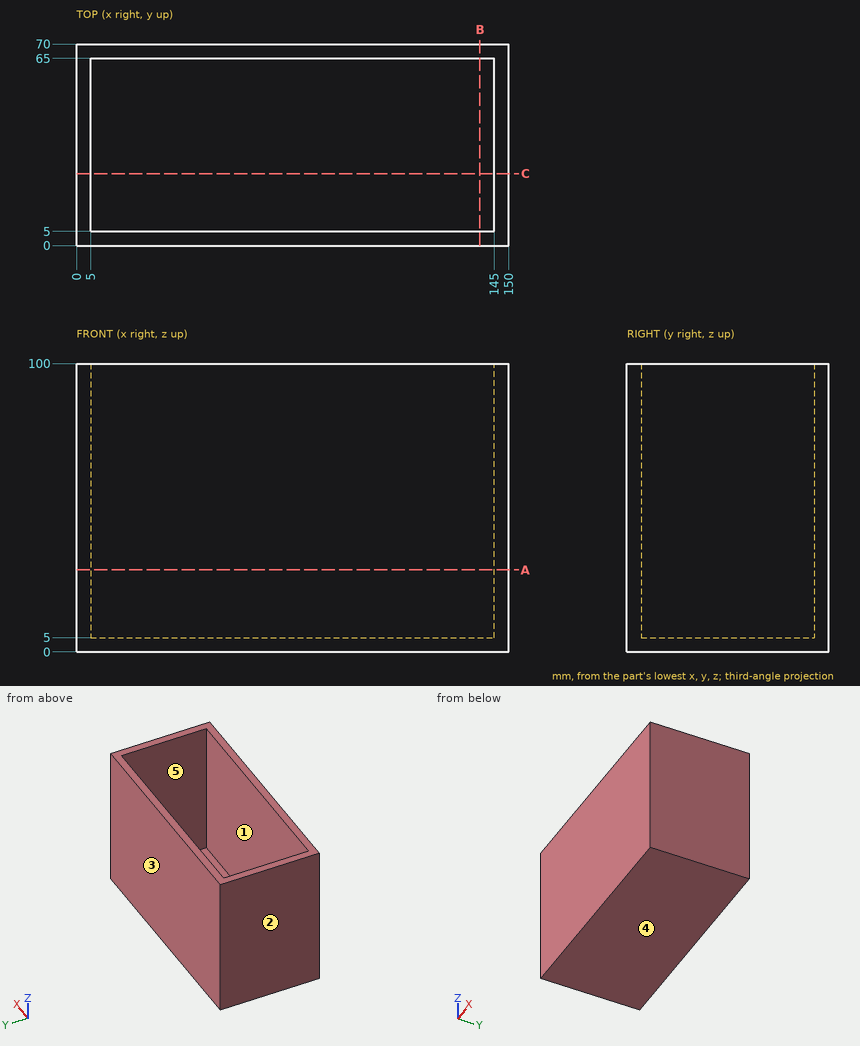
Geometry check sheet. Reference: drawing and pictorial views, mm from the part's lowest x, y, z. A direction names the side the tool comes from. Round coordinates to 2 decimals unless told otherwise and drop trailing zeros. Loops run counter-clockwise (first coordinate to the right, second up) from the corner with the lowest first, then second, coordinate; pieces in that order, holes last.
1. Gauge pin test, flat ends, axial feed: pin 1 Ø10 at (x, y) = (24.5, 17.5) entering from +Z; pin 2 Ø1.5 at (y, z) = (16, 27) entering from -X. Record the tip position at first contact, or that the pin passes through.
2. Scan lines: probe 1 along Y at (x, z) = (118, 37.5); probe 2 along X at (y, z) = (31, 77); probe 3 along Z at (x, y) = (95.5, 28). Record each from-to range of solid material in increasing order.
3. Mould release check, pull along X, two halves, no side actions. Record for the marked faces 1, 2 and 3: released by +X, released by -X, zero draft, split by the parting line, or undercut.
4. Sectioned sample at A-A on z = 28.5. Record the boundary of the cut face in (x, y), and give its area (3 significant figures).
5. Sectioned sample at B-B on x = 140. Record the boundary of the cut face in (y, z).
6. Set-up check for the marked faces 4 and 5: record each of +Z, -Z, +X, -X, +Y, -Y from which the full face is reachable in a straight line by a thin tool's end or side.
7. Sectioned sample at C-C on y = 25. Record the boundary of the cut face in (x, z).
Recorded:
1. pin 1: stops at z = 5
1. pin 2: stops at x = 0
2. probe 1: y = 0 to 5, 65 to 70
2. probe 2: x = 0 to 5, 145 to 150
2. probe 3: z = 0 to 5
3. face 1: undercut
3. face 2: released by -X
3. face 3: zero draft
4. outline: (0, 0) - (150, 0) - (150, 70) - (0, 70) - close; hole (5, 5) - (145, 5) - (145, 65) - (5, 65) - close
4. area: 2,100 mm2
5. outline: (0, 0) - (70, 0) - (70, 100) - (65, 100) - (65, 5) - (5, 5) - (5, 100) - (0, 100) - close
6. face 4: -Z, +X, -X, +Y, -Y
6. face 5: +Z
7. outline: (0, 0) - (150, 0) - (150, 100) - (145, 100) - (145, 5) - (5, 5) - (5, 100) - (0, 100) - close
